CAD build for the part. Positions are in the model's coordinates, mm. Face numbers are marked on the shaded views. Give positions to 0.01 mm unless a question says otherwise; leave off trailing zeros. Order: outer loops, then holes, each group sorted by start corner. A loop starts at its lowest first (then second) coordinate and runs counter-clockwise, first axis right, second up. Notation, with made-up numbers: (-23, 79.5) -> (30, 79.5) arc R31 cw to (30, 116.5) -> close; hole circle Ø3 at (43.5, 51). An arc over 180 degrees is marked (long way). Use one line per item in the form item = value. Start each with the question number.
1) Cut at B-B, the plane y = 11. Give the cut face in (x, z), and give its area (3 significant figures).
2) Cut at C-C, the plane x = 0. Give the cut face in (y, z).
3) Cut at D-D, the plane z = 0. Give the cut face in (x, y).
4) Cut at A-A, the plane y = -7. Give the cut face in (x, z).
5) Mould opens along Z. For the marked faces 1, 2, 3 and 4 say: pulls with the +Z half, pulls with the -Z half, needs draft (parallel to the pull), parting line crosses it, or undercut.
6) Drop flat-ended pins along their axis: P1, Ø1, axis at x = 11.5, z = -13.5, coming from the -Y side; P2, Ø1, axis at y = -22, z = -27, coming from the -X side; P3, Ø4, axis at x = 8, y = -5.5, coming from the +Z side. Give the stop position or say it passes through.
7) Probe line 1 (Z direction, x = 6, y = -5); line 2 (X direction, y = -34.5, z = 0); line 3 (Y direction, x = -21, z = -12). List the from-to ranges inside material, lowest first.
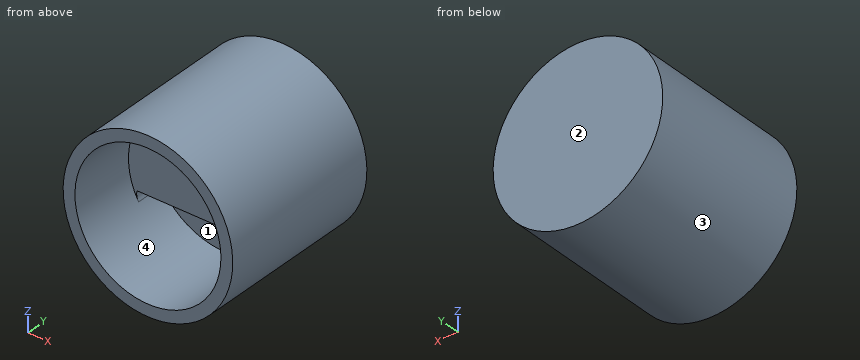
from build123d import *

# Parameters (mm, degrees)
SKETCH1_R           = 39.5
BOSS_EXTRUDE1_DEPTH = 33.9
BOSS_EXTRUDE3_DEPTH = 13.7
BOSS_EXTRUDE4_START = -44.7
SKETCH7_R           = 39.5
SKETCH7_R_2         = 34
BOSS_EXTRUDE4_DEPTH = 44.7
SKETCH8_R           = 8
SKETCH8_R_2         = 2.75
SKETCH8_R_3         = 4.9
CUT_EXTRUDE2_DEPTH  = 19


with BuildPart() as part:
    # Sketch1 → Boss-Extrude1 (new body)
    with BuildSketch(Plane(origin=(0, 0, 0), x_dir=(1, 0, 0), z_dir=(0, 1, 0))):
        with Locations(Location((0, 0, 0), (0, 0, 270))):
            Circle(SKETCH1_R)
    extrude(amount=BOSS_EXTRUDE1_DEPTH)

    # Sketch6 → Boss-Extrude3 (add)
    with BuildSketch(Plane(origin=(0, 0, 0), x_dir=(1, 0, 0), z_dir=(0, 1, 0))):
        with BuildLine():
            Line((29.737090224, 12.56), (-29.737090224, 12.56))
            ThreePointArc((-29.737090224, 12.56), (-29.806512789, 14.933347645), (-29, 17.166537216))
            ThreePointArc((-29, 17.166537216), (-33.7, 0), (-29, -17.166537216))
            ThreePointArc((-29, -17.166537216), (-29.806512789, -14.933347645), (-29.737090224, -12.56))
            Line((-29.737090224, -12.56), (29.737090224, -12.56))
            ThreePointArc((29.737090224, -12.56), (29.806512789, -14.933347645), (29, -17.166537216))
            ThreePointArc((29, -17.166537216), (33.7, 0), (29, 17.166537216))
            ThreePointArc((29, 17.166537216), (29.806512789, 14.933347645), (29.737090224, 12.56))
        make_face()
    extrude(amount=-BOSS_EXTRUDE3_DEPTH)

    # Sketch7 → Boss-Extrude4 (add)
    with BuildSketch(Plane(origin=(0, 0, 0), x_dir=(1, 0, 0), z_dir=(0, 1, 0)).offset(BOSS_EXTRUDE4_START)):
        with Locations(Location((0, 0, 0), (0, 0, 270))):
            Circle(SKETCH7_R)
        with Locations(Location((0, 0, 0), (0, 0, 270))):
            Circle(SKETCH7_R_2, mode=Mode.SUBTRACT)
    extrude(amount=BOSS_EXTRUDE4_DEPTH)

    # Sketch8 → Cut-Extrude2 (cut)
    with BuildSketch(Plane(origin=(0, 0, 0), x_dir=(1, 0, 0), z_dir=(0, 1, 0))):
        with Locations(Location((0, -23.44, 0), (0, 0, 270))):
            Circle(SKETCH8_R)
        with Locations(Location((12.5, -26.56, 0), (0, 0, 270))):
            Circle(SKETCH8_R_2)
        with Locations(Location((20, -19.06, 0), (0, 0, 270))):
            Circle(SKETCH8_R_3)
        with Locations(Location((-12.5, -26.56, 0), (0, 0, 90))):
            Circle(SKETCH8_R_2)
        with Locations(Location((-20, -19.06, 0), (0, 0, 90))):
            Circle(SKETCH8_R_3)
    extrude(amount=CUT_EXTRUDE2_DEPTH, mode=Mode.SUBTRACT)


solid = part.part
Result:
q1.outline = circle Ø79 at (0, 0); hole circle Ø9.8 at (-20, 19.06); hole circle Ø5.5 at (-12.5, 26.56); hole circle Ø16 at (0, 23.44); hole circle Ø5.5 at (12.5, 26.56); hole circle Ø9.8 at (20, 19.06)
q1.area = 4,500 mm²
q2.outline = (-44.7, -39.5) -> (33.9, -39.5) -> (33.9, 39.5) -> (-44.7, 39.5) -> (-44.7, 34) -> (0, 34) -> (0, 31.44) -> (19, 31.44) -> (19, 15.44) -> (0, 15.44) -> (0, 12.56) -> (-13.7, 12.56) -> (-13.7, -12.56) -> (0, -12.56) -> (0, -34) -> (-44.7, -34) -> close
q3.outline = (-39.5, -44.7) -> (-34, -44.7) -> (-34, 0) -> (-33.7, 0) -> (-33.7, -13.7) -> (33.7, -13.7) -> (33.7, 0) -> (34, 0) -> (34, -44.7) -> (39.5, -44.7) -> (39.5, 33.9) -> (-39.5, 33.9) -> close
q4.outline = circle Ø79 at (0, 0); (-29.74, -12.56) -> (29.74, -12.56) arc R6.36 cw to (29, -17.17) arc R33.7 ccw to (29, 17.17) arc R6.36 cw to (29.74, 12.56) -> (-29.74, 12.56) arc R6.36 cw to (-29, 17.17) arc R33.7 ccw to (-29, -17.17) arc R6.36 cw to start; hole circle Ø68 at (0, 0)
q5.face_1 = undercut
q5.face_2 = needs draft
q5.face_3 = parting line crosses it
q5.face_4 = undercut
q6.P1 = 0
q6.P2 = -29.29
q6.P3 = 39.04
q7.line_1 = -39.04 to -33.47, -12.56 to 12.56, 33.47 to 39.04
q7.line_2 = -39.5 to -34, 34 to 39.5
q7.line_3 = -13.7 to 33.9
